Build history of the part. All positions in model axes, mm. Give positions to 0.01 mm unless a question says otherwise; leave off trailing zeros. Loops run counter-clockwise (first coordinate to the right, second up) from the corner with the lowest first, then second, coordinate; pieces in that order, holes last. Notation, with made-up numbers: M 57.25,12 L 112.25,12 A19 cw 112.25,16 Z; hole C 13,-29 d3. An arc over 180 degrees is marked long. Put each result on its own line as item: value.
```python
from build123d import *


with BuildPart() as part:
    # Sketch1 → Revolve1 (revolve)
    with BuildSketch(Plane(origin=(0, 0, 0), x_dir=(0, 0, -1), z_dir=(1, 0, 0))):
        Polygon((-4.409523218, 7.4), (-4.409523218, 8.5), (-1.909523218, 8.5), (-1.909523218, 3.5), (-4.409523218, 3.5), (-4.409523218, 4.25), (-4.409523218, 6.15), (-6.409523218, 6.15), (-6.409523218, 7.4), align=None)
    revolve(axis=Axis((0, 0, 52.974875508), (0, 0, -1)))


solid = part.part
```
Q1. Mould opens along X. For faces 1 (the cylindrical face through (-7.224, -1.604, 5.396)), 2 (the cylindrical face through (-6.004, -1.333, 5.424)), 3 (the flat face through (-3, 3, 4.41)), 4 (the flat face through (7, 3, 4.41)) say: pulls with the +X half, pulls with the -X half, needs draft (parallel to the pull), parting line crosses it, or undercut.
Here are the results:
face 1: parting line crosses it
face 2: undercut
face 3: undercut
face 4: needs draft
Q2. Probe line 1 (X direction, y = 0, z = 5.35); line 2 (X direction, y = -0.5, z = 3.7); line 3 (Z direction, x = 7, y = 2.75). List the from-to ranges inside material, lowest first. Write a range as from..to.
Here are the results:
line 1: -7.4..-6.15, 6.15..7.4
line 2: -8.49..-3.46, 3.46..8.49
line 3: 1.91..4.41
Q3. Slice it at D-D (y = 4.75). List the corners of the cut face in (x, z).
Here are the results:
outline: M -7.05,1.91 L 7.05,1.91 L 7.05,4.41 L 5.67,4.41 L 5.67,6.41 L 3.91,6.41 L 3.91,4.41 L -3.91,4.41 L -3.91,6.41 L -5.67,6.41 L -5.67,4.41 L -7.05,4.41 Z
Q4. Drop flat-ended pins along their axis: pin 1 Ø5 at (x, y) = (1.5, -1) entering from +Z; pin 2 Ø2 at (x, y) = (-0.5, -1) entering from -Z; pin 3 Ø2 at (y, z) = (4, 4) entering from +X. Give the stop position or say it passes through.
Here are the results:
pin 1: z = 4.41
pin 2: through
pin 3: x = 7.95
Q5. Slice it at C-C (z = 2.9). List the corners of the cut face in (x, y), and give its area (3 significant figures).
Here are the results:
outline: C 0,0 d17; hole C 0,0 d7
area: 188 mm²
Q6. Slice it at A-A (y = 0). List the corners of the cut face in (x, z), and give its area (3 significant figures).
Here are the results:
outline: M -8.5,1.91 L -3.5,1.91 L -3.5,4.41 L -6.15,4.41 L -6.15,6.41 L -7.4,6.41 L -7.4,4.41 L -8.5,4.41 Z; M 3.5,1.91 L 8.5,1.91 L 8.5,4.41 L 7.4,4.41 L 7.4,6.41 L 6.15,6.41 L 6.15,4.41 L 3.5,4.41 Z
area: 30.0 mm²
